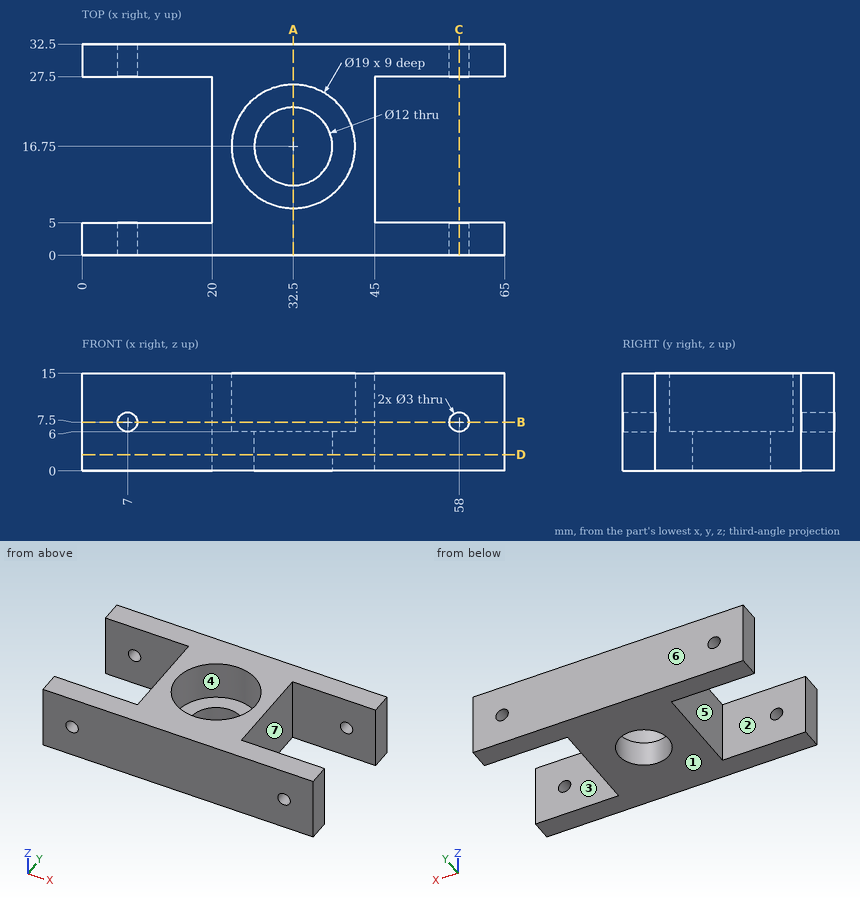
Geometry check sheet. Reference: drawing and pictorial views, mm from the part's lowest x, y, z. A direction names the side the tool comes from. Coordinates: 2 decimals unless noted, no trailing zeros. Order: outer loops, then holes, each group sorted by start corner. A loop starts at its lowest first (then second) coordinate and runs counter-clockwise, first axis right, second up.
Item 1: Tool access check on the marked faces 1, 2 and 3. Record the directions out of +Z, -Z, +X, -X, +Y, -Y that give a thin tool (end or side, any length) a straight path to the whole face; none if there is none.
Item 2: Section check A-A (x = 32.5). Enter the section's corners in (y, z), plus the area to 4 significant figures.
Item 3: Mould release check, pull along X, two halves, no side actions. Record for the marked faces 4, 5, 6 and 7: released by +X, released by -X, zero draft, split by the parting line, or undercut.
Item 4: Scan lines: line 1 along X through (y, z) = (1.05, 7.5); line 2 along Y through (x, z) = (15.5, 13.5); line 3 along X through (y, z) = (16.5, 9). Record each from-to range of solid material in increasing order.
Item 5: Section check B-B (z = 7.5). Count the separate pieces of the cut face and the enclosed holes in it, plus the area to 3 significant figures.
Item 6: Depth check by flat-ended pin: pin 1 (6 mm diameter, centred on y = 22, z = 8, fed in from +X); pin 2 (5 mm diameter, centred on y = 18.5, z = 13, fed in from -X); pin 3 (5.5 mm diameter, centred on x = 30.5, y = 14, fed in from +Z). Enter the tip coordinate at first touch or a pass-through.
Item 7: Section check C-C (x = 58). Enter the section's corners in (y, z).
Item 8: Section check D-D (z = 2.5). Enter the section's corners in (x, y).
Check sheet entries:
1. face 1: -Z, +X, -X, +Y, -Y
1. face 2: +Z, -Z, -X
1. face 3: +Z, -Z, +X
2. outline: (0, 0) - (10.75, 0) - (10.75, 6) - (7.25, 6) - (7.25, 15) - (0, 15) - close; (22.75, 0) - (32.5, 0) - (32.5, 15) - (26.25, 15) - (26.25, 6) - (22.75, 6) - close
2. area: 244.5 mm2
3. face 4: undercut
3. face 5: released by -X
3. face 6: zero draft
3. face 7: released by +X
4. line 1: x = 0 to 5.5, 8.5 to 56.5, 59.5 to 65
4. line 2: y = 0 to 5, 27.5 to 32.5
4. line 3: x = 20 to 23, 42 to 45
5. separate pieces: 5
5. enclosed holes: 1
5. area: 869 mm2
6. pin 1: stops at x = 45
6. pin 2: stops at x = 20
6. pin 3: stops at z = 6
7. outline: (0, 0) - (5, 0) - (5, 6) - (0, 6) - close; (0, 9) - (5, 9) - (5, 15) - (0, 15) - close; (27.5, 0) - (32.5, 0) - (32.5, 6) - (27.5, 6) - close; (27.5, 9) - (32.5, 9) - (32.5, 15) - (27.5, 15) - close
8. outline: (0, 0) - (65, 0) - (65, 5) - (45, 5) - (45, 27.5) - (65, 27.5) - (65, 32.5) - (0, 32.5) - (0, 27.5) - (20, 27.5) - (20, 5) - (0, 5) - close; hole circle Ø12 at (32.5, 16.75)
